Could you check a few things on this model? Use its own coordinates, in mm. Give positions to 0.01 mm unless a question says otherwise; leave off trailing zeros. One line per question, with ' | ' between items.
from build123d import *

# Parameters (mm, degrees)
SKETCH2_W               = 215
SKETCH2_H               = 139.732878208
BOSS_EXTRUDE1_DEPTH     = 10
SKETCH3_R               = 2.04999698
SKETCH3_R_2             = 2.049996201
SKETCH3_R_3             = 2.049998036
SKETCH3_R_4             = 2.05000301
SKETCH3_R_5             = 2.05000489
SKETCH3_R_6             = 2.05000167
SKETCH3_R_7             = 2.049998726
SKETCH3_R_8             = 2.050000522
SKETCH3_R_9             = 2.050000228
SKETCH3_R_10            = 2.050000557
SKETCH3_R_11            = 2.050001917
SKETCH3_R_12            = 2.050001502
CUT_EXTRUDE2_DEPTH      = 11
CUT_EXTRUDE2_DEPTH_BACK = 1


with BuildPart() as part:
    # Sketch2 → Boss-Extrude1 (new body)
    with BuildSketch(Plane(origin=(0, 0, 0), x_dir=(1, 0, 0), z_dir=(0, 1, 0))):
        with Locations((107.5, -70)):
            Rectangle(SKETCH2_W, SKETCH2_H)
    extrude(amount=BOSS_EXTRUDE1_DEPTH)

    # Sketch3 → Cut-Extrude2 (cut, two sides)
    with BuildSketch(Plane(origin=(0, 0, 0), x_dir=(1, 0, 0), z_dir=(0, 1, 0))) as cut_extrude2_sk:
        with Locations((20.000003077, -129.000001764)):
            Circle(SKETCH3_R)
        with Locations((74.999999742, -129.000001144)):
            Circle(SKETCH3_R_2)
        with Locations((130.000001864, -128.999997495)):
            Circle(SKETCH3_R_3)
        with Locations((172.961008424, -125.432773785)):
            Circle(SKETCH3_R_4)
        with Locations((202.661132812, -91.812960049)):
            Circle(SKETCH3_R_5)
        with Locations((202.661143569, -48.187042941)):
            Circle(SKETCH3_R_6)
        with Locations((172.961008675, -14.567229705)):
            Circle(SKETCH3_R_7)
        with Locations((130.000001694, -10.999999378)):
            Circle(SKETCH3_R_8)
        with Locations((75.000000263, -10.999999084)):
            Circle(SKETCH3_R_9)
        with Locations((20.000004874, -11.000001196)):
            Circle(SKETCH3_R_10)
        with Locations((10.999999837, -47.000000994)):
            Circle(SKETCH3_R_11)
        with Locations((11.000000285, -93.0000014)):
            Circle(SKETCH3_R_12)
    extrude(amount=CUT_EXTRUDE2_DEPTH, mode=Mode.SUBTRACT)
    extrude(cut_extrude2_sk.sketch, amount=-CUT_EXTRUDE2_DEPTH_BACK, mode=Mode.SUBTRACT)


solid = part.part
Q1. If I drill on line 1 along Z through (x, y) = (130.5, 9); line 2 along Z through (x, y) = (201.5, 3.75); line 3 along X through (y, z) = (0.5, 12), over which ranges is the centre line in solid material (lowest first)?
Answer below:
line 1: z = 0.13 to 9.01, 12.99 to 127.01, 130.99 to 139.87 | line 2: z = 0.13 to 46.5, 49.88 to 90.12, 93.5 to 139.87 | line 3: x = 0 to 18.21, 21.79 to 73.21, 76.79 to 128.21, 131.79 to 215
Q2. Will these pins go through, and if not, where does the flat tip stop? pin 1 (5.5 mm diameter, centred on x = 130, z = 129, fed in from +Y); pin 2 (3.5 mm diameter, centred on x = 172.96, z = 14.57, fed in from -Y).
Answer below:
pin 1: stops at y = 10 | pin 2: passes through
Q3. If we mould it in two halves opening along Z, with no side actions, what happens to faces 1 (the flat face through (106, 0, 69)), 2 (the cylindrical face through (19.556, 4.93, 131.001)), 3 (the flat face through (106, 5, 0.134)), 4 (the cylindrical face through (128.5, 4.9, 127.6))? For each: +Z half, -Z half, draft (parallel to the pull), parting line (faces both ways), or undercut.
Answer below:
face 1: draft | face 2: undercut | face 3: -Z half | face 4: undercut
